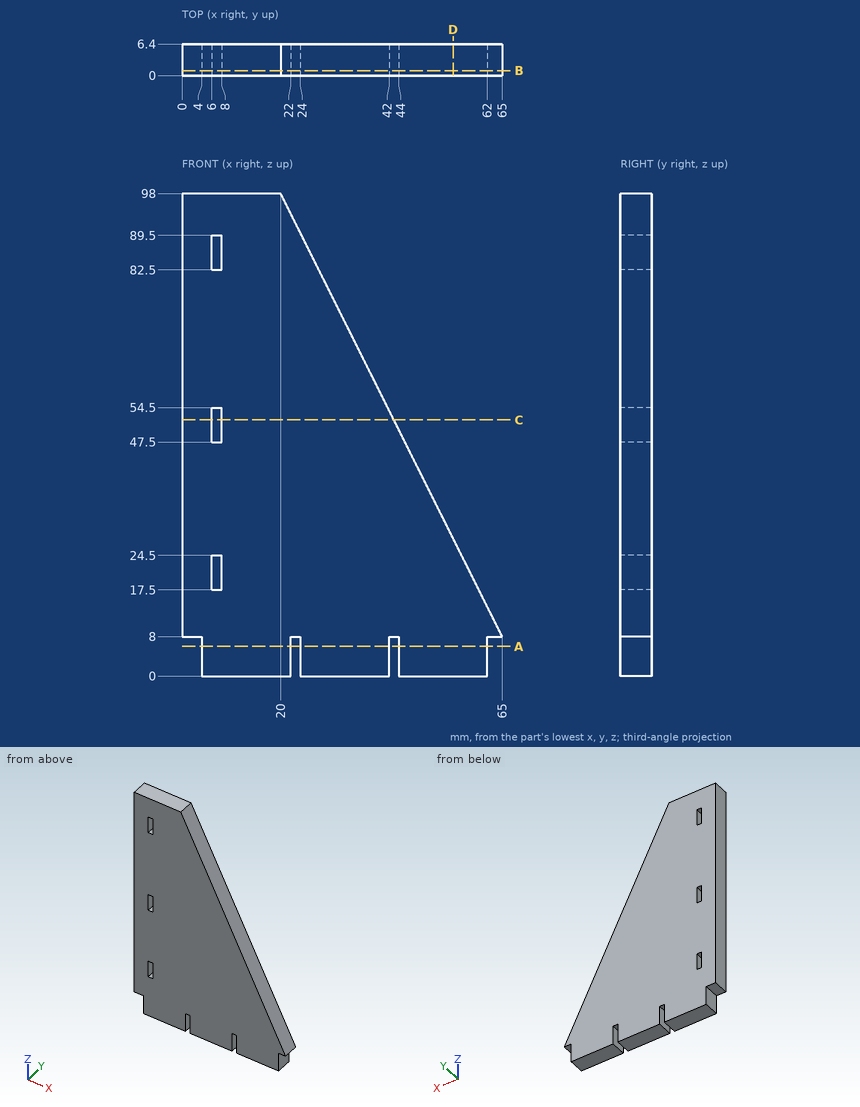
The figure shows three views and two pictorial views of one solid part (mm, origin at its lowest corner). Answer the questions. Round coordinates to 2 decimals unless told otherwise and drop trailing zeros. Order: outer loops, then holes, each group sorted by start corner. A loop starts at its lowest first (then second) coordinate and runs counter-clockwise, first axis right, second up. Notation, with made-up numbers: (75, 34) - (98, 34) arc R23 ccw to (98, 70) - close; hole circle Ø9 at (-21.75, -2). An arc over 180 degrees is marked (long way). Write item = value, one per line. Start each with the question number.
1) Straight lines are drawn through the part: L1, parallel to X at y = 1, z = 6.5; L2, parallel to Z at x = 6.5, y = 2.5; L3, parallel to Z at x = 57, y = 1.25. For each, find the intervals that lie inside material, in ascending order.
2) Section B-B, the plane y = 1 is taken. Write down the section's boundary in (x, z).
3) Section A-A, the plane z = 6 is taken. Write down the section's boundary in (x, y).
4) Section C-C, the plane z = 52 is taken. Write down the section's boundary in (x, y), plus the area to 3 significant figures.
5) Given pin 1 (3 mm diameter, centred on y = 4, z = 86.5, fed in from -X); pin 2 (3 mm diameter, centred on y = 5, z = 51, fed in from +X); pin 3 (1 mm diameter, centred on x = 23, y = 4.5, fed in from -Z); pin 4 (3 mm diameter, centred on y = 4, z = 3.5, fed in from -X), each flat-ended and moving along its own axis, determine where each tip first touches the part or whether it passes through.
6) Section D-D, the plane x = 55 is taken. Write down the section's boundary in (y, z), plus the area to 3 significant figures.
Results list:
q1.L1 = 4 to 22, 24 to 42, 44 to 62
q1.L2 = 0 to 17.5, 24.5 to 47.5, 54.5 to 82.5, 89.5 to 98
q1.L3 = 0 to 24
q2.outline = (0, 8) - (4, 8) - (4, 0) - (22, 0) - (22, 8) - (24, 8) - (24, 0) - (42, 0) - (42, 8) - (44, 8) - (44, 0) - (62, 0) - (62, 8) - (65, 8) - (20, 98) - (0, 98) - close; hole (6, 17.5) - (8, 17.5) - (8, 24.5) - (6, 24.5) - close; hole (6, 47.5) - (8, 47.5) - (8, 54.5) - (6, 54.5) - close; hole (6, 82.5) - (8, 82.5) - (8, 89.5) - (6, 89.5) - close
q3.outline = (4, 0) - (22, 0) - (22, 6.4) - (4, 6.4) - close; (24, 0) - (42, 0) - (42, 6.4) - (24, 6.4) - close; (44, 0) - (62, 0) - (62, 6.4) - (44, 6.4) - close
q4.outline = (0, 0) - (6, 0) - (6, 6.4) - (0, 6.4) - close; (8, 0) - (43, 0) - (43, 6.4) - (8, 6.4) - close
q4.area = 262 mm^2
q5.pin_1 = 0
q5.pin_2 = 44.25
q5.pin_3 = 8
q5.pin_4 = 4
q6.outline = (0, 0) - (6.4, 0) - (6.4, 28) - (0, 28) - close
q6.area = 179 mm^2
